Geometry: final body of the model. Coordinates: model frame, mm. A direction names the side the tool comes from. Round coordinates to 2 decimals unless told otherwise and drop trailing zeros. Write each loop counter-clockwise with the first axis right and the second up, starting at its lowest first coordinate (ties: lowest second). Pieces come first, ordered by that corner, then holes.
from build123d import *

# Parameters (mm, degrees)
F0_W     = 50
F0_H     = 50
F1_DEPTH = 1
F2_W     = 50
F2_H     = 50
F3_DEPTH = 1
F5_DEPTH = 1
F7_DEPTH = 1


with BuildPart() as f1:
    # F0 (on Top) → F1 (new body)
    with BuildSketch(Plane.XY):
        Rectangle(F0_W, F0_H)
    extrude(amount=F1_DEPTH)

    # F2 (on face) → F3 (join)
    with BuildSketch(Plane.XZ.offset(25)):
        with Locations((0, 25)):
            Rectangle(F2_W, F2_H)
    extrude(amount=F3_DEPTH)

    # F4 (on face) → F5 (cut)
    with BuildSketch(Plane.XZ.offset(26)):
        with BuildLine():
            Line((15.5, 40.5), (13.75, 40.5))
            ThreePointArc((13.75, 40.5), (14.2625631329, 39.2625631329), (15.5, 38.75))
            Line((15.5, 38.75), (15.5, 40.5))
        make_face()
        with BuildLine():
            ThreePointArc((17.25, 40.5), (15.5, 42.25), (13.75, 40.5))
            Line((13.75, 40.5), (15.5, 40.5))
            Line((15.5, 40.5), (15.5, 38.75))
            ThreePointArc((15.5, 38.75), (16.7374368671, 39.2625631329), (17.25, 40.5))
        make_face()
        with BuildLine():
            ThreePointArc((-15.5, 38.75), (-14.2625631329, 39.2625631329), (-13.75, 40.5))
            Line((-13.75, 40.5), (-15.5, 40.5))
            Line((-15.5, 40.5), (-15.5, 38.75))
        make_face()
        with BuildLine():
            Line((-15.5, 40.5), (-13.75, 40.5))
            ThreePointArc((-13.75, 40.5), (-16.7374368671, 41.7374368671), (-15.5, 38.75))
            Line((-15.5, 38.75), (-15.5, 40.5))
        make_face()
        with BuildLine():
            Line((15.5, 9.5), (15.5, 11.25))
            ThreePointArc((15.5, 11.25), (14.2625631329, 10.7374368671), (13.75, 9.5))
            Line((13.75, 9.5), (15.5, 9.5))
        make_face()
        with BuildLine():
            ThreePointArc((17.25, 9.5), (16.7374368671, 10.7374368671), (15.5, 11.25))
            Line((15.5, 11.25), (15.5, 9.5))
            Line((15.5, 9.5), (13.75, 9.5))
            ThreePointArc((13.75, 9.5), (15.5, 7.75), (17.25, 9.5))
        make_face()
        with BuildLine():
            ThreePointArc((-13.75, 9.5), (-14.2625631329, 10.7374368671), (-15.5, 11.25))
            Line((-15.5, 11.25), (-15.5, 9.5))
            Line((-15.5, 9.5), (-13.75, 9.5))
        make_face()
        with BuildLine():
            Line((-15.5, 9.5), (-15.5, 11.25))
            ThreePointArc((-15.5, 11.25), (-16.7374368671, 8.2625631329), (-13.75, 9.5))
            Line((-13.75, 9.5), (-15.5, 9.5))
        make_face()
        with BuildLine():
            Line((0, 13.95), (0, 36.05))
            ThreePointArc((0, 36.05), (-11.05, 25), (0, 13.95))
        make_face()
        with BuildLine():
            ThreePointArc((11.05, 25), (7.8135299321, 32.8135299321), (0, 36.05))
            Line((0, 36.05), (0, 13.95))
            ThreePointArc((0, 13.95), (7.8135299321, 17.1864700679), (11.05, 25))
        make_face()
    extrude(amount=-F5_DEPTH, mode=Mode.SUBTRACT)

    # F6 (on face) → F7 (cut)
    with BuildSketch(Plane.XY.offset(1)):
        with BuildLine():
            Line((-15, 12.95), (-15, 15))
            Line((-15, 15), (-17.05, 15))
            ThreePointArc((-17.05, 15), (-16.4495689014, 13.5504310986), (-15, 12.95))
        make_face()
        with BuildLine():
            Line((-12.95, 15), (-15, 15))
            Line((-15, 15), (-15, 12.95))
            ThreePointArc((-15, 12.95), (-13.5504310986, 13.5504310986), (-12.95, 15))
        make_face()
        with BuildLine():
            Line((-15, -15), (-15, -12.95))
            ThreePointArc((-15, -12.95), (-16.4495689014, -13.5504310986), (-17.05, -15))
            Line((-17.05, -15), (-15, -15))
        make_face()
        with BuildLine():
            ThreePointArc((-12.95, -15), (-13.5504310986, -13.5504310986), (-15, -12.95))
            Line((-15, -12.95), (-15, -15))
            Line((-15, -15), (-12.95, -15))
        make_face()
        with BuildLine():
            Line((15, 15), (12.95, 15))
            ThreePointArc((12.95, 15), (13.5504310986, 13.5504310986), (15, 12.95))
            Line((15, 12.95), (15, 15))
        make_face()
        with BuildLine():
            Line((17.05, 15), (15, 15))
            Line((15, 15), (15, 12.95))
            ThreePointArc((15, 12.95), (16.4495689014, 13.5504310986), (17.05, 15))
        make_face()
        with BuildLine():
            ThreePointArc((15, -12.95), (13.5504310986, -13.5504310986), (12.95, -15))
            Line((12.95, -15), (15, -15))
            Line((15, -15), (15, -12.95))
        make_face()
        with BuildLine():
            ThreePointArc((17.05, -15), (16.4495689014, -13.5504310986), (15, -12.95))
            Line((15, -12.95), (15, -15))
            Line((15, -15), (17.05, -15))
        make_face()
        with BuildLine():
            ThreePointArc((17.05, 15), (15, 17.05), (12.95, 15))
            Line((12.95, 15), (15, 15))
            Line((15, 15), (17.05, 15))
        make_face()
        with BuildLine():
            Line((15, -15), (12.95, -15))
            ThreePointArc((12.95, -15), (15, -17.05), (17.05, -15))
            Line((17.05, -15), (15, -15))
        make_face()
        with BuildLine():
            Line((-17.05, 15), (-15, 15))
            Line((-15, 15), (-12.95, 15))
            ThreePointArc((-12.95, 15), (-15, 17.05), (-17.05, 15))
        make_face()
        with BuildLine():
            Line((-12.95, -15), (-15, -15))
            Line((-15, -15), (-17.05, -15))
            ThreePointArc((-17.05, -15), (-15, -17.05), (-12.95, -15))
        make_face()
        with BuildLine():
            Line((-15, -12.95), (-15, 12.95))
            ThreePointArc((-15, 12.95), (-16.4495689014, 13.5504310986), (-17.05, 15))
            Line((-17.05, 15), (-17.1, 15))
            Line((-17.1, 15), (-17.1, -15))
            Line((-17.1, -15), (-17.05, -15))
            ThreePointArc((-17.05, -15), (-16.4495689014, -13.5504310986), (-15, -12.95))
        make_face()
        with BuildLine():
            Line((17.1, 15), (17.05, 15))
            ThreePointArc((17.05, 15), (16.4495689014, 13.5504310986), (15, 12.95))
            Line((15, 12.95), (15, -12.95))
            ThreePointArc((15, -12.95), (16.4495689014, -13.5504310986), (17.05, -15))
            Line((17.05, -15), (17.1, -15))
            Line((17.1, -15), (17.1, 15))
        make_face()
        with BuildLine():
            Line((-12.9, 15), (-12.95, 15))
            ThreePointArc((-12.95, 15), (-13.5504310986, 13.5504310986), (-15, 12.95))
            Line((-15, 12.95), (-15, -12.95))
            ThreePointArc((-15, -12.95), (-13.5504310986, -13.5504310986), (-12.95, -15))
            Line((-12.95, -15), (-12.9, -15))
            Line((-12.9, -15), (-12.9, 15))
        make_face()
        with BuildLine():
            Line((12.95, 15), (12.9, 15))
            Line((12.9, 15), (12.9, -15))
            Line((12.9, -15), (12.95, -15))
            ThreePointArc((12.95, -15), (13.5504310986, -13.5504310986), (15, -12.95))
            Line((15, -12.95), (15, 12.95))
            ThreePointArc((15, 12.95), (13.5504310986, 13.5504310986), (12.95, 15))
        make_face()
    extrude(amount=-F7_DEPTH, mode=Mode.SUBTRACT)


solid = f1.part
1) Section D-D on x = 20. Output: boundary loops of the cut face in (y, z).
2) Section C-C on z = 15. Output: boundary loops of the cut face in (x, y), plus the area to 3 significant figures.
3) First-contact query: P1, Ø1, axis at x = 9.5, y = -15, coming from the +Z side. Flat tip, straight axial feed; report the tip coordinate or a pass-through.
4) Line query: probe 1 along X at (y, z) = (-25.5, 40.5); probe 2 along Z at (x, y) = (-15.5, -25.4); probe 3 along Y at (x, z) = (-1, 40). Output: solid intervals per line, ascending.
5) Section B-B on x = -7. Output: boundary loops of the cut face in (y, z), plus the area to 3 significant figures.
6) Draft query along X for faces 1 (the cylindrical face through (15.05, 17.05, 0.51)), 2 (the flat face through (-25, -0.4, 0.8)), 3 (the flat face through (0, 0, 1)). Return one class per face: pulls with the +X half, pulls with the -X half, needs draft (parallel to the pull), parting line crosses it, or undercut.
7) Reachability of faces 4 (the flat face through (25, -0.4, 0.8)), 5 (the cylindrical face through (-15.05, -17.05, 0.51)), 6 (the flat face through (0, -25, 37)) from +Z, -Z, +X, -X, +Y, -Y: full face, straight path, thin tool, end or side. Return the list, or none.
8) Section A-A on y = -5. Output: boundary loops of the cut face in (x, z).
Filled in:
1. outline: (-26, 0) - (25, 0) - (25, 1) - (-25, 1) - (-25, 50) - (-26, 50) - close
2. outline: (-25, -26) - (-4.7, -26) - (-4.7, -25) - (-25, -25) - close; (4.7, -26) - (25, -26) - (25, -25) - (4.7, -25) - close
2. area: 40.6 mm2
3. P1: stops at z = 1
4. probe 1: x = -25 to -17.25, -13.75 to 13.75, 17.25 to 25
4. probe 2: z = 0 to 7.75, 11.25 to 38.75, 42.25 to 50
4. probe 3: y = -26 to -25
5. outline: (-26, 0) - (25, 0) - (25, 1) - (-25, 1) - (-25, 16.45) - (-26, 16.45) - close; (-26, 33.55) - (-25, 33.55) - (-25, 50) - (-26, 50) - close
5. area: 82.9 mm2
6. face 1: undercut
6. face 2: pulls with the -X half
6. face 3: needs draft
7. face 4: +Z, -Z, +X, +Y, -Y
7. face 5: +Z, -Z
7. face 6: +Z, +X, -X, +Y
8. outline: (-25, 0) - (-17.1, 0) - (-17.1, 1) - (-25, 1) - close; (-12.9, 0) - (12.9, 0) - (12.9, 1) - (-12.9, 1) - close; (17.1, 0) - (25, 0) - (25, 1) - (17.1, 1) - close
